```python
from build123d import *

# Parameters (mm, degrees)
SKETCH093_R             = 6.5
SKETCH093_R_2           = 2.5
PAD050_DEPTH            = 6
SKETCH094_R             = 5
SKETCH094_R_2           = 2.522437
PAD051_DEPTH            = 7
SKETCH095_R             = 6.5
SKETCH095_R_2           = 2.522437
PAD052_DEPTH            = 1
SKETCH096_R             = 1
PAD053_DEPTH            = 7
BODY035_ROLL_ANGLE      = 135
BODY035_PLACEMENT_ANGLE = 180
SKETCH100_R             = 15
PAD054_DEPTH            = 8.5
POCKET031_DEPTH         = 2.5
POLARPATTERN023_COUNT   = 4
SKETCH097_R             = 1
HOLE008_DEPTH           = 25
POLARPATTERN022_COUNT   = 4
SKETCH098_R             = 4
POCKET030_DEPTH         = 6.001
BODY036_PLACEMENT_ANGLE = 90
SKETCH102_R             = 8
POCKET032_DEPTH         = 8.501


with BuildPart() as polea007:
    # Sketch093 → Pad050 (new body)
    with BuildSketch(Plane.YZ):
        Circle(SKETCH093_R)
        Circle(SKETCH093_R_2, mode=Mode.SUBTRACT)
    extrude(amount=PAD050_DEPTH)

    # Sketch094 (on Face3 of Pad050) → Pad051 (join)
    with BuildSketch(Plane(origin=(0, 0, 0), x_dir=(0, 1, 0), z_dir=(-1, 0, 0))):
        Circle(SKETCH094_R)
        Circle(SKETCH094_R_2, mode=Mode.SUBTRACT)
    extrude(amount=PAD051_DEPTH)

    # Sketch095 (on Face6 of Pad051) → Pad052 (join)
    with BuildSketch(Plane(origin=(-7, 0, 0), x_dir=(0, 1, 0), z_dir=(-1, 0, 0))):
        Circle(SKETCH095_R)
        Circle(SKETCH095_R_2, mode=Mode.SUBTRACT)
    extrude(amount=PAD052_DEPTH)

    # Sketch096 → Pad053 (join)
    with BuildSketch(Plane.XZ):
        with Locations((3, 0)):
            Circle(SKETCH096_R)
    extrude(amount=PAD053_DEPTH)


with BuildPart() as polea007_1:
    # Body035 roll: moved
    add(polea007.part.rotate(Axis((0, 0, 0), (1, 0, 0)), BODY035_ROLL_ANGLE))


with BuildPart() as polea007_2:
    # Body035 placement: moved
    add(polea007_1.part.rotate(Axis((0, 0, 0), (0, 0, 1)), BODY035_PLACEMENT_ANGLE))


with BuildPart() as body037:
    # Sketch100 → Pad054 (new body)
    with BuildSketch(Plane.XY):
        Circle(SKETCH100_R)
    extrude(amount=PAD054_DEPTH)

    # Sketch099 (on Face3 of Pad054) → Pocket031 (cut)
    with BuildSketch(Plane.XY.offset(8.5)):
        with BuildLine():
            ThreePointArc((-5.26869, 1.578261), (0, -5.5), (5.26869, 1.578261))
            Line((2.107476, 12.131304), (5.26869, 1.578261))
            ThreePointArc((2.107476, 12.131304), (0, 13.7), (-2.107476, 12.131304))
            Line((-2.107476, 12.131304), (-5.26869, 1.578261))
        make_face()
    pocket031 = extrude(amount=-POCKET031_DEPTH, mode=Mode.SUBTRACT)

    # PolarPattern023: Pocket031 ×4 about axis
    polarpattern023_axis = Axis((0, 0, 8.5), (0, 0, 1))
    for i in range(1, POLARPATTERN023_COUNT):
        add(pocket031.rotate(polarpattern023_axis, i * 360 / POLARPATTERN023_COUNT), mode=Mode.SUBTRACT)

    # Sketch097 (on Face21 of PolarPattern023) → Hole008 (cut)
    with BuildSketch(Plane.XY.offset(6)):
        with Locations((0, 11)):
            Circle(SKETCH097_R)
    hole008 = extrude(amount=-HOLE008_DEPTH, mode=Mode.SUBTRACT)

    # PolarPattern022: Hole008 ×4 about axis
    polarpattern022_axis = Axis((0, 0, 6), (0, 0, 1))
    for i in range(1, POLARPATTERN022_COUNT):
        add(hole008.rotate(polarpattern022_axis, i * 360 / POLARPATTERN022_COUNT), mode=Mode.SUBTRACT)

    # Sketch098 (on Face25 of PolarPattern022) → Pocket030 (cut, through all)
    with BuildSketch(Plane.XY.offset(6)):
        Circle(SKETCH098_R)
    extrude(amount=-POCKET030_DEPTH, mode=Mode.SUBTRACT)


with BuildPart() as body037_1:
    # Body036 placement: moved
    add(body037.part.moved(Location((0, 0, 0))).rotate(Axis((0, 0, 0), (0, -1, 0)), BODY036_PLACEMENT_ANGLE))

    # Cut006: cut polea007
    add(polea007_2.part, mode=Mode.SUBTRACT)

    # Sketch102 (on Face3 of BaseFeature006) → Pocket032 (cut, through all)
    with BuildSketch(Plane(origin=(-8.5, 0, 0), x_dir=(0, -1, 0), z_dir=(-1, 0, 0))):
        Circle(SKETCH102_R)
    extrude(amount=-POCKET032_DEPTH, mode=Mode.SUBTRACT)


solid = body037_1.part
```
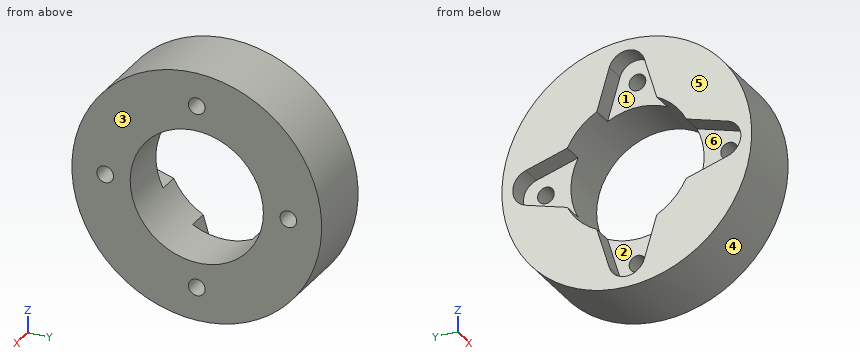
Read the model definition and answer for the solid it produces. Units are mm, in the model's axes. Face numbers are marked on the shaded views. A direction names the side the tool comes from. Give positions to 0.01 mm unless a question says otherwise; leave off trailing zeros. Loops run counter-clockwise (first coordinate to the right, second up) from the corner with the lowest first, then second, coordinate; pieces in that order, holes last.
Item 1: The part is cut by section D-D (z = 4). Write down the section's boundary in (x, y), and give its area (3 significant figures).
Item 2: The part is cut by section A-A (x = -7.25). Write down the section's boundary in (y, z).
Item 3: The part is cut by section C-C (y = 11). Write down the section's boundary in (x, z), and give its area (3 significant figures).
Item 4: The part is cut by section B-B (z = 0). Write down the section's boundary in (x, y), and give its area (3 significant figures).
Item 5: Find the intervals of material crossed by line 1 along Y through (x, z) = (-3.75, -9); line 2 along Z through (x, y) = (-3.7, -11); line 3 along Y through (x, z) = (-6.75, 10.25), in increasing order.
Item 6: For the marked faces 5 and 6, determine the directions among +Z, -Z, +X, -X, +Y, -Y from which every point of the face is accessible in a straight line to the end or side of a thin tool.
Item 7: The mould has two halves that part along Z. Classify the marked faces 1, 2, 3 and 4: released by +Z, released by -Z, zero draft, split by the parting line, or undercut.
Item 8: Each of these flat-tipped pins is pushed along its axis until it touches: pin 1 Ø13 at (y, z) = (0, 0) entering from -X; pin 2 Ø3 at (y, z) = (0, -11) entering from +X; pin 3 Ø2 at (x, z) = (-3, 8) entering from -Y; pin 4 Ø2 at (y, z) = (-9.5, 1.5) entering from -X. Where does it stop, or does it pass through?
Taken from the geometry:
1. outline: (-8.5, -14.46) - (0, -14.46) - (0, -6.93) - (-8.5, -6.93) - close; (-8.5, 6.93) - (0, 6.93) - (0, 14.46) - (-8.5, 14.46) - close
1. area: 128 mm2
2. outline: circle Ø30 at (0, 0); hole (-12.13, -2.11) - (-7.14, -3.6) arc R8 ccw to (-3.6, -7.14) - (-2.11, -12.13) arc R2.2 ccw to (2.11, -12.13) - (3.6, -7.14) arc R8 ccw to (7.14, -3.6) - (12.13, -2.11) arc R2.2 ccw to (12.13, 2.11) - (7.14, 3.6) arc R8 ccw to (3.6, 7.14) - (2.11, 12.13) arc R2.2 ccw to (-2.11, 12.13) - (-3.6, 7.14) arc R8 ccw to (-7.14, 3.6) - (-12.13, 2.11) arc R2.2 ccw to start
3. outline: (-8.5, -10.2) - (0, -10.2) - (0, -1) - (-6, -1) - (-6, -2.45) - (-8.5, -2.45) - close; (-8.5, 2.45) - (-6, 2.45) - (-6, 1) - (0, 1) - (0, 10.2) - (-8.5, 10.2) - close
3. area: 149 mm2
4. outline: (-8.5, -15) - (0, -15) - (0, -12) - (-6, -12) - (-6, -13.7) - (-8.5, -13.7) - close; (-8.5, 13.7) - (-6, 13.7) - (-6, 12) - (0, 12) - (0, 15) - (-8.5, 15) - close; (-6, -10) - (0, -10) - (0, -8) - (-6, -8) - close; (-6, 8) - (0, 8) - (0, 10) - (-6, 10) - close
4. area: 66.5 mm2
5. line 1: y = -12 to 12
5. line 2: z = -10.2 to -1, 1 to 10.2
5. line 3: y = -10.95 to -2.67, 2.67 to 10.95
6. face 5: +Z, -Z, -X, +Y, -Y
6. face 6: -X
7. face 1: undercut
7. face 2: undercut
7. face 3: zero draft
7. face 4: split by the parting line
8. pin 1: passes through
8. pin 2: stops at x = 0
8. pin 3: stops at y = -13.27
8. pin 4: stops at x = -6
